The figure shows three views and two pictorial views of one solid part (mm, origin at its lowest corner). Answer the questions. Round coordinates to 2 decimals unless told otherwise and drop trailing zeros. Write each loop counter-clockwise with the first axis right and the second up, starting at its lowest first coordinate (ties: lowest second). Pieces come first, ordered by that corner, then holes.
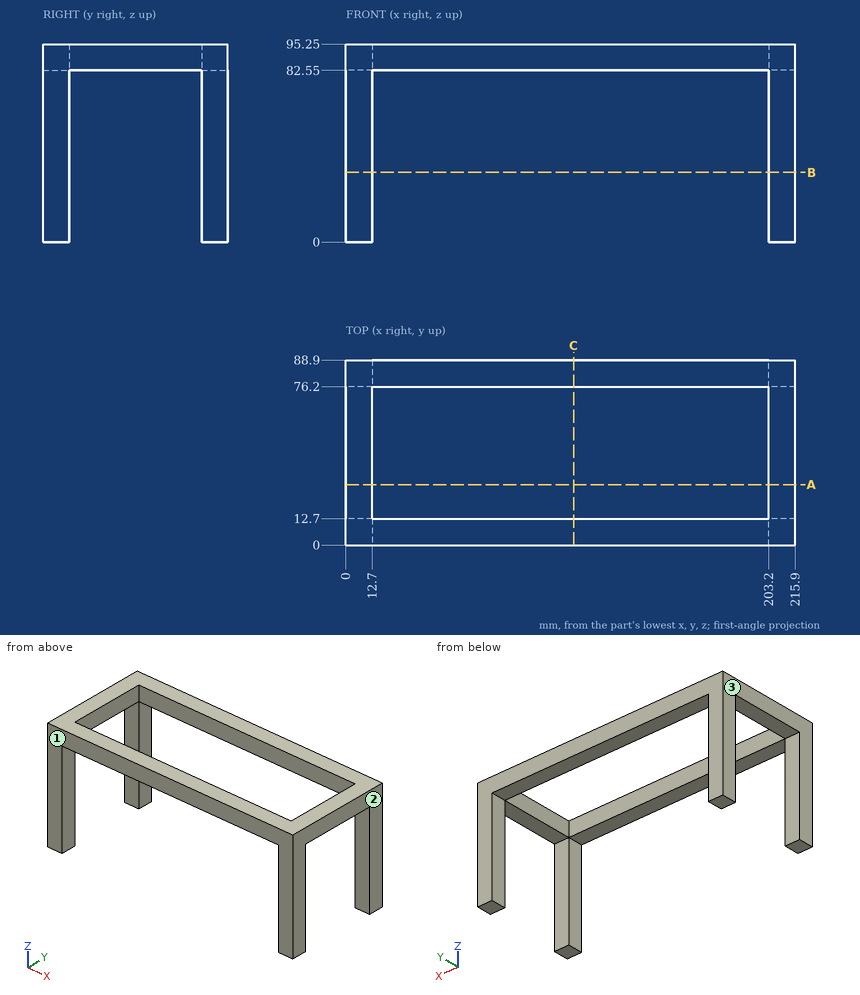
Q1. Section C-C (x = 109.5) is taken. Determine the outline of the cut face in (y, z), then the cut area to 3 significant figures.
Verdict:
outline: (0, 82.55) - (12.7, 82.55) - (12.7, 95.25) - (0, 95.25) - close; (76.2, 82.55) - (88.9, 82.55) - (88.9, 95.25) - (76.2, 95.25) - close
area: 323 mm2
Q2. Section B-B (z = 33.5) is taken. Determine the outline of the cut face in (x, y).
Verdict:
outline: (0, 0) - (12.7, 0) - (12.7, 12.7) - (0, 12.7) - close; (0, 76.2) - (12.7, 76.2) - (12.7, 88.9) - (0, 88.9) - close; (203.2, 0) - (215.9, 0) - (215.9, 12.7) - (203.2, 12.7) - close; (203.2, 76.2) - (215.9, 76.2) - (215.9, 88.9) - (203.2, 88.9) - close
Q3. Straight lines are drawn through the part: probe 1 along X at (y, z) = (7, 75.5); probe 2 along Y at (x, z) = (147.5, 85); probe 3 along Z at (x, y) = (147.5, 11). For each, find the intervals that lie inside material, in ascending order.
Verdict:
probe 1: x = 0 to 12.7, 203.2 to 215.9
probe 2: y = 0 to 12.7, 76.2 to 88.9
probe 3: z = 82.55 to 95.25
Q4. Determine the mould class of the marked faces 1, 2 and 3 for opening direction X: pulls with the +X half, pulls with the -X half, needs draft (parallel to the pull), parting line crosses it, or undercut.
Verdict:
face 1: needs draft
face 2: pulls with the +X half
face 3: pulls with the -X half
Q5. Flat-ended cylindrical pins translate along their axes: pin 1 Ø6.5 at (x, y) = (147, 3.5) entering from -Z; pin 2 Ø2 at (x, y) = (111, 74) entering from +Z. Find the tip coordinate at first contact, or state that the pin passes through.
Verdict:
pin 1: stops at z = 82.55
pin 2: passes through
Q6. Section A-A (y = 29) is taken. Determine the outline of the cut face in (x, z), then the cut area to 3 significant figures.
Verdict:
outline: (0, 82.55) - (12.7, 82.55) - (12.7, 95.25) - (0, 95.25) - close; (203.2, 82.55) - (215.9, 82.55) - (215.9, 95.25) - (203.2, 95.25) - close
area: 323 mm2
